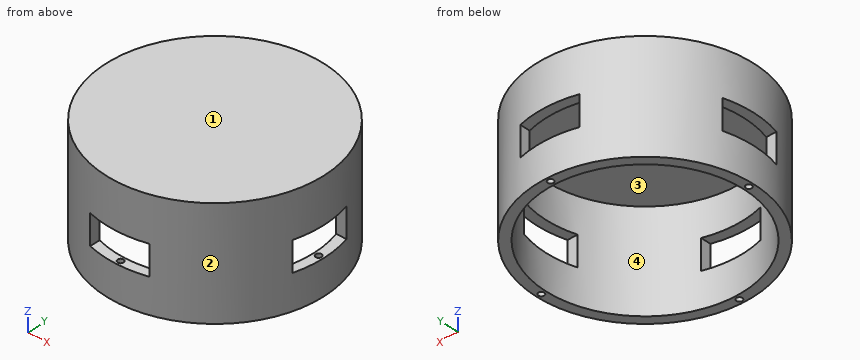
Autodesk Inventor part; units mm, degrees
ref_plane "YZ Plane" through (0, 0, 0) normal (1, 0, 0) x (0, 1, 0)
ref_plane "XZ Plane" through (0, 0, 0) normal (0, 1, 0) x (-1, 0, 0)
ref_plane "XY Plane" through (0, 0, 0) normal (0, 0, 1) x (1, 0, 0)
sketch "Sketch1" plane through (0, 0, 0) normal (0, 0, 1) x (1, 0, 0)
  circle A0 centre (0, 0) radius 55
  circle A1 centre (0, 0) radius 50
  circle A2 centre (0, 52.5) radius 1.5
  circle A3 centre (-52.5, 0) radius 1.5
  circle A4 centre (0, -52.5) radius 1.5
  circle A5 centre (52.5, 0) radius 1.5
  dimension "d2" = 110
  dimension "d3" = 100
  dimension "d4" = 3
  dimension "d5" = 0
  dimension "d6" = 52.5
  dimension "d7" = 360
extrude "Extrusion1" add sketch "Sketch1" along normal blind 5 contours A0 | A1
extrude "Extrusion2" add sketch "Sketch1" against normal blind 50
extrude "Extrusion3" add sketch "Sketch1" along normal mid plane 10 contours A2 | A3 | A4 | A5
sketch "Sketch2" plane through (0, 0, 0) normal (0, 1, 0) x (-1, 0, 0)
  line L0 (-15, -17.5) -> (15, -17.5)
  line L1 (15, -17.5) -> (15, -32.5)
  line L2 (15, -32.5) -> (-15, -32.5)
  line L3 (-15, -32.5) -> (-15, -17.5)
  line L4 (-15, -17.5) -> (15, -32.5) construction
  line L5 (15, -17.5) -> (-15, -32.5) construction
  point P0 (0, 0)
  point P1 (0, -25)
  dimension "d14" = 0
  dimension "d15" = 25
  dimension "d16" = 30
  dimension "d17" = 15
extrude "Extrusion4" cut sketch "Sketch2" along normal through all both and the other way through all
pattern_circular "Circular Pattern1" count 3 over 180 about axis through (0, 0, 0) along (0, 0, -1) of "Extrusion4"
extrude "Extrusion5" add sketch "Sketch1" against normal blind 17.5 contours A2 | A3 | A4 | A5
equation "\"d2\" = Diameter"
properties part number "Base"
Check sheet for the modelled part. Datum: model origin and axes. Units: mm. Face numbers are marked on the shaded views. Coordinates: 2 decimals unless noted, no trailing zeros. Order: outer loops, then holes, each group sorted by start corner. A loop starts at its lowest first (then second) coordinate and runs counter-clockwise, first axis right, second up. Notation, with made-up numbers: M 56.25,22 L 65.25,22 A16 ccw 65.25,27 Z; hole C 27.5,-4 d3. An arc over 180 degrees is marked long. One line per question, with ' | ' between items. Start each with the question number.
Item 1: Sectioned sample at B-B on z = -20. Record the cut outline in (x, y), and give its area (3 significant figures).
Item 2: Mould release check, pull along X, two halves, no side actions. Record for the marked faces 1, 2, 3 and 4: pulls with the +X half, pulls with the -X half, needs draft (parallel to the pull), parting line crosses it, or undercut.
Item 3: Sectioned sample at C-C on x = 10. Record the cut outline in (y, z).
Item 4: Sectioned sample at A-A on y = 0. Record the cut outline in (x, z), and give its area (3 significant figures).
Item 5: Gauge pin test, flat ends, axial feed: P1, Ø8, axis at x = 43, z = -35, coming from the +Y side; P2, Ø8, axis at x = 29.5, y = -7.5, coming from the -Z side; P3, Ø3.5, axis at x = 0, y = -52.5, coming from the -Z side; P4, Ø4, axis at x = -49.5, z = -27, coming from the -Y side. Record the tip position at first contact, or that the pin passes through.
Item 6: Sectioned sample at D-D on z = -10.5. Record the cut outline in (x, y), and give its area (3 significant figures).
Item 7: Material ranges on line 1 (Y direction, x = 0, z = -41); line 2 (Z direction, x = 38, y = 20); line 3 (Y direction, x = 32.5, z = -13), recorded low to high.
Answer below:
1) outline: M -52.92,-15 A55 ccw -15,-52.92 L -15,-47.7 A50 cw -47.7,-15 Z; M -52.92,15 L -47.7,15 A50 cw -15,47.7 L -15,52.92 A55 ccw Z; M 15,-52.92 A55 ccw 52.92,-15 L 47.7,-15 A50 cw 15,-47.7 Z; M 15,47.7 A50 cw 47.7,15 L 52.92,15 A55 ccw 15,52.92 Z | area: 1,040 mm^2
2) face 1: needs draft | face 2: parting line crosses it | face 3: undercut | face 4: undercut
3) outline: M -54.08,-50 L -48.99,-50 L -48.99,-32.5 L -54.08,-32.5 Z; M -54.08,-17.5 L -48.99,-17.5 L -48.99,0 L 48.99,0 L 48.99,-17.5 L 54.08,-17.5 L 54.08,5 L -54.08,5 Z; M 48.99,-50 L 54.08,-50 L 54.08,-32.5 L 48.99,-32.5 Z
4) outline: M -55,-50 L -54,-50 L -54,-32.5 L -55,-32.5 Z; M -55,-17.5 L -50,-17.5 L -50,0 L 50,0 L 50,-17.5 L 55,-17.5 L 55,5 L -55,5 Z; M -51,-50 L -50,-50 L -50,-32.5 L -51,-32.5 Z; M 50,-50 L 51,-50 L 51,-32.5 L 50,-32.5 Z; M 54,-50 L 55,-50 L 55,-32.5 L 54,-32.5 Z | area: 795 mm^2
5) P1: stops at y = 38.78 | P2: stops at z = 0 | P3: stops at z = -50 | P4: stops at y = -27.73
6) outline: C 0,0 d110; hole C 0,0 d100 | area: 1,650 mm^2
7) line 1: y = -55 to -54, -51 to -50, 50 to 51, 54 to 55 | line 2: z = 0 to 5 | line 3: y = -44.37 to -38, 38 to 44.37
